The model under review builds one solid part; all positions refer to its coordinate system, in mm. Face numbers are marked on the shaded views. A direction names the side the tool comes from. Round coordinates to 2 decimals unless told otherwise and drop trailing zeros. Loops run counter-clockwise (first coordinate to the right, second up) from the corner with the lowest first, then second, coordinate; pieces in that order, holes last. Notation, with made-up numbers: M 48,60 L 96,60 A18 ccw 96,87 Z; hole C 30.5,35.5 d1. An arc over 180 degrees is marked long. Answer as a JSON object with one key per item and string values. Group by question number.
Item 1: Consider section C-C (z = -6.5). Give the boundary of the cut face in (x, y), and give its area (3 significant figures).
Item 2: Consider section D-D (y = 25.5). Give the boundary of the cut face in (x, z).
Item 3: Insertion check: P1, Ø8, axis at x = -8.5, z = 8.5, coming from the +Y side; P2, Ø0.6, axis at x = 0, z = 6.5, coming from the +Y side; P3, Ø3, axis at x = 0, y = 25, coming from the +Z side. Each pin has a flat end and moves straight along its axis. Give the tip position at first contact, or say it passes through.
Item 4: Consider section B-B (y = 13.5). Give the boundary of the cut face in (x, z), and give its area (3 significant figures).
Item 5: Tool access review of the marked faces 1, 2 and 3: name each direction out of +Z, -Z, +X, -X, +Y, -Y from which nothing blocks a thin tool from reaching the whole face with its end or side.
Item 6: To check wall thickness, follow line 1 (X direction, y = 18.7, z = 0); line 2 (Y direction, x = -9, z = 1.75); line 3 (Y direction, x = 15.5, z = -1.75). State the ranges of each line that lie inside material, in increasing order.
Item 7: The part is to be moulded in two halves that separate along Z. For the marked faces 4, 5, 6 and 7, say which applies: +Z half, -Z half, draft (parallel to the pull), parting line (faces both ways), or undercut.
Item 8: Consider section A-A (x = 0). Give the boundary of the cut face in (y, z), and give its area (3 significant figures).
```python
from build123d import *

# Parameters (mm, degrees)
SKETCH1_R           = 14
BOSS_EXTRUDE1_DEPTH = 19.22
SKETCH2_W           = 41.795845618
SKETCH2_H           = 7
BOSS_EXTRUDE2_DEPTH = 0.84
FILLET2_R           = 3.5
SKETCH3_R           = 2
CUT_EXTRUDE1_DEPTH  = 0.84
SKETCH4_R           = 4.58
BOSS_EXTRUDE3_DEPTH = 1.64
SKETCH5_R           = 2.5
BOSS_EXTRUDE4_DEPTH = 8.26
SKETCH6_OUTSIDE_W   = 55.422
SKETCH6_OUTSIDE_H   = 41.626
SKETCH6_OUTSIDE_W_2 = 6.15537624
SKETCH6_OUTSIDE_H_2 = 2.88
CUT_EXTRUDE2_DEPTH  = 6.2


with BuildPart() as part:
    # Sketch1 → Boss-Extrude1 (new body)
    with BuildSketch(Plane(origin=(0, 0, 0), x_dir=(1, 0, 0), z_dir=(0, 1, 0))):
        with Locations(Location((0, 0, 0), (0, 0, 270))):
            Circle(SKETCH1_R)
    extrude(amount=BOSS_EXTRUDE1_DEPTH)

    # Sketch2 → Boss-Extrude2 (add)
    with BuildSketch(Plane(origin=(0, 19.22, 0), x_dir=(1, 0, 0), z_dir=(0, 1, 0))):
        with Locations((0, -0.294656178)):
            Rectangle(SKETCH2_W, SKETCH2_H)
    extrude(amount=-BOSS_EXTRUDE2_DEPTH)

    # Fillet2
    fillet2_edges = [part.edges().sort_by_distance(p)[0] for p in [
        (20.897922809, 18.8, -3.205343822),
        (20.897922809, 18.8, 3.794656178),
        (-20.897922809, 18.8, -3.205343822),
        (-20.897922809, 18.8, 3.794656178),
    ]]
    fillet(fillet2_edges, radius=FILLET2_R - 0.0001)  # a hair under: the kernel refuses the full size

    # Sketch3 → Cut-Extrude1 (cut)
    with BuildSketch(Plane(origin=(0, 19.22, 0), x_dir=(1, 0, 0), z_dir=(0, 1, 0))):
        with Locations(Location((-16.94163256, 0, 0), (0, 0, 270))):
            Circle(SKETCH3_R)
        with Locations(Location((16.94163256, 0, 0), (0, 0, 90))):
            Circle(SKETCH3_R)
    extrude(amount=-CUT_EXTRUDE1_DEPTH, mode=Mode.SUBTRACT)

    # Sketch4 → Boss-Extrude3 (add)
    with BuildSketch(Plane(origin=(0, 19.22, 0), x_dir=(1, 0, 0), z_dir=(0, 1, 0))):
        with Locations(Location((0, -8.213475026, 0), (0, 0, 270))):
            Circle(SKETCH4_R)
    extrude(amount=BOSS_EXTRUDE3_DEPTH)

    # Sketch5 → Boss-Extrude4 (add)
    with BuildSketch(Plane(origin=(0, 20.86, 0), x_dir=(1, 0, 0), z_dir=(0, 1, 0))):
        with Locations(Location((0, -8.213475026, 0), (0, 0, 270))):
            Circle(SKETCH5_R)
    extrude(amount=BOSS_EXTRUDE4_DEPTH)

    # Sketch6 outside → Cut-Extrude2 (cut)
    with BuildSketch(Plane(origin=(0, 29.12, 0), x_dir=(1, 0, 0), z_dir=(0, 1, 0))):
        Rectangle(SKETCH6_OUTSIDE_W, SKETCH6_OUTSIDE_H)
        with Locations((0, -8.278567721)):
            Rectangle(SKETCH6_OUTSIDE_W_2, SKETCH6_OUTSIDE_H_2, mode=Mode.SUBTRACT)
    extrude(amount=-CUT_EXTRUDE2_DEPTH, mode=Mode.SUBTRACT)


solid = part.part
```
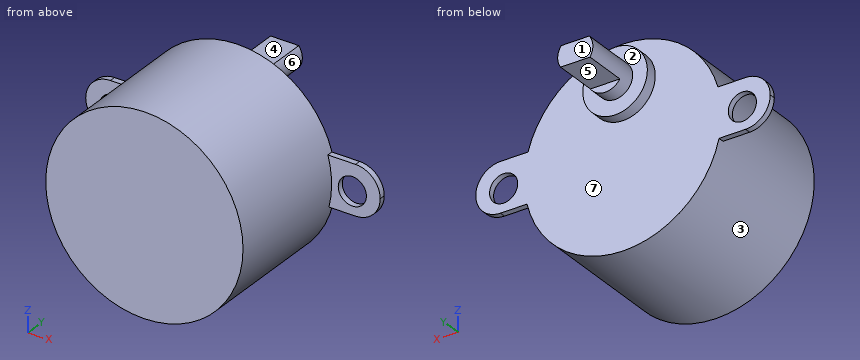
Geometry results:
{
 "1": {"outline": "M -12.4,0 L 12.4,0 L 12.4,19.22 L -12.4,19.22 Z", "area": "477 mm^2"},
 "2": {"outline": "M -2.09,6.84 L 2.09,6.84 A2.5 ccw 2,9.72 L -2,9.72 A2.5 ccw Z"},
 "3": {"P1": "stops at y = 20.86", "P2": "stops at y = 22.92", "P3": "stops at z = 9.72"},
 "4": {"outline": "C 0,0 d28", "area": "616 mm^2"},
 "5": {"face 1": "+Z, -Z, +X, -X, +Y", "face 2": "+Y", "face 3": "-Y"},
 "6": {"line 1": "x = -20.89 to -18.94, -14.94 to 14.94, 18.94 to 20.89", "line 2": "y = 0 to 19.22", "line 3": "y = 18.38 to 19.22"},
 "7": {"face 4": "+Z half", "face 5": "-Z half", "face 6": "parting line", "face 7": "draft"},
 "8": {"outline": "M 0,-14 L 19.22,-14 L 19.22,3.63 L 20.86,3.63 L 20.86,5.71 L 22.92,5.71 L 22.92,6.84 L 29.12,6.84 L 29.12,9.72 L 22.92,9.72 L 22.92,10.71 L 20.86,10.71 L 20.86,12.79 L 19.22,12.79 L 19.22,14 L 0,14 Z", "area": "581 mm^2"}
}
